The figure shows three views and two pictorial views of one solid part (mm, origin at its lowest corner). Answer the questions. A direction names the side the tool comes from. Coordinates: 2 decimals unless noted, no trailing zeros. Loops run counter-clockwise (first coordinate to the right, second up) from the corner with the lowest first, then second, coordinate; pieces in that order, holes last.
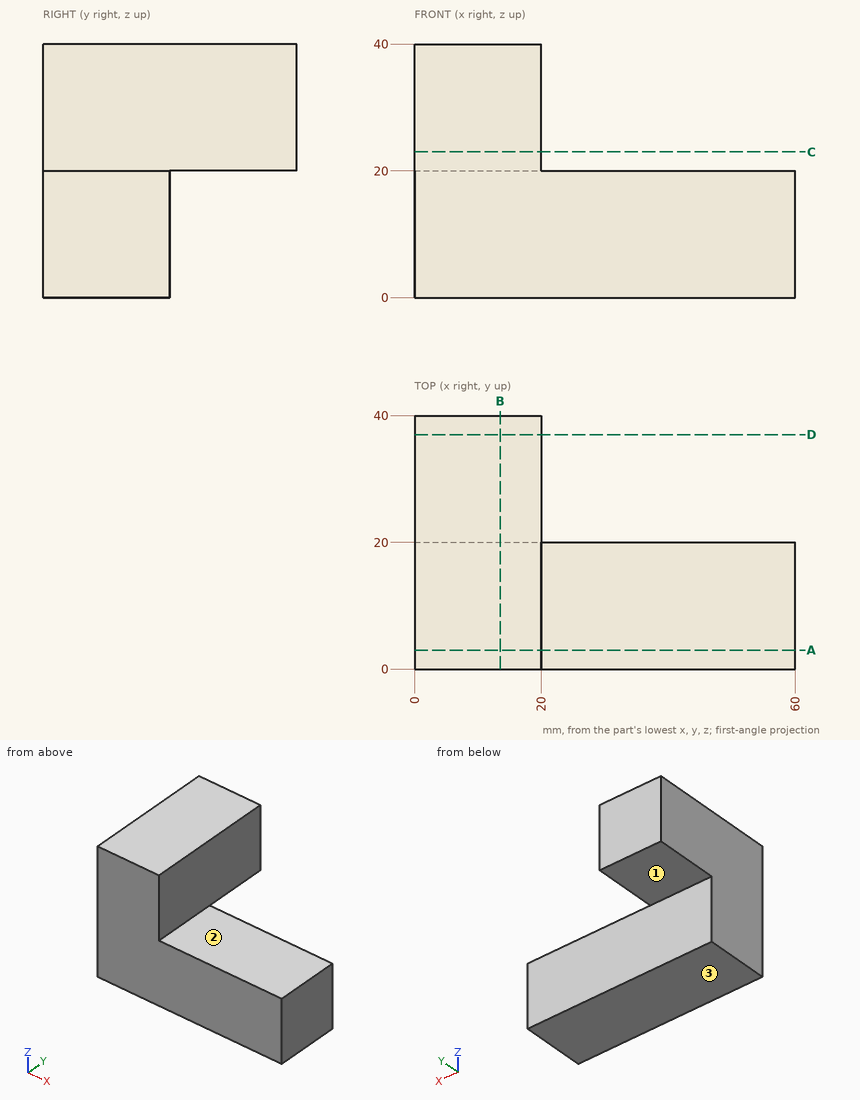
Q1. A cutting plane is placed at A-A (y = 3). Give the vertices of the cut face in (x, z), then the cut area to 3 significant figures.
Findings below:
outline: (0, 0) - (60, 0) - (60, 20) - (20, 20) - (20, 40) - (0, 40) - close
area: 1,600 mm2
Q2. Flat-ended cylindrical pins translate along their axes: pin 1 Ø3 at (y, z) = (18, 34) entering from +X; pin 2 Ø8 at (x, y) = (10, 26.5) entering from -Z; pin 3 Ø12 at (x, y) = (53.5, 14.5) entering from +Z; pin 4 Ø2 at (y, z) = (6.5, 35.5) entering from -X. Find the tip coordinate at first contact, or state that the pin passes through.
Findings below:
pin 1: stops at x = 20
pin 2: stops at z = 20
pin 3: stops at z = 20
pin 4: stops at x = 0
Q3. A cutting plane is placed at C-C (z = 23). Give the vertices of the cut face in (x, y), then the cut area to 3 significant figures.
Findings below:
outline: (0, 0) - (20, 0) - (20, 40) - (0, 40) - close
area: 800 mm2
Q4. A cutting plane is placed at B-B (x = 13.5). Give the vertices of the cut face in (y, z), then the cut area to 3 significant figures.
Findings below:
outline: (0, 0) - (20, 0) - (20, 20) - (40, 20) - (40, 40) - (0, 40) - close
area: 1,200 mm2
Q5. A cutting plane is placed at D-D (y = 37). Give the vertices of the cut face in (x, z).
Findings below:
outline: (0, 20) - (20, 20) - (20, 40) - (0, 40) - close
Q6. Which of the six approach directions +Z, -Z, +X, -X, +Y, -Y give full straight-line access (tool end or side, diameter ignored) to the marked faces 1, 2 and 3?
Findings below:
face 1: -Z, +X, -X, +Y
face 2: +Z, +X, +Y, -Y
face 3: -Z, +X, -X, +Y, -Y
Q7. A straight line is drawn through the part: probe 1 along X at (y, z) = (22.5, 30.5). Find the intervals that lie inside material, in ascending order.
Findings below:
probe 1: x = 0 to 20
